Drawing for the job (mm, zero at the part's lowest x, y, z). Give positions to 0.01 mm unless a question says otherwise; leave off trailing zeros. Write each loop counter-clockwise with the first axis right and the second up, starting at its lowest first coordinate (ties: lowest second). Pieces come first, ordered by that corner, then holes.
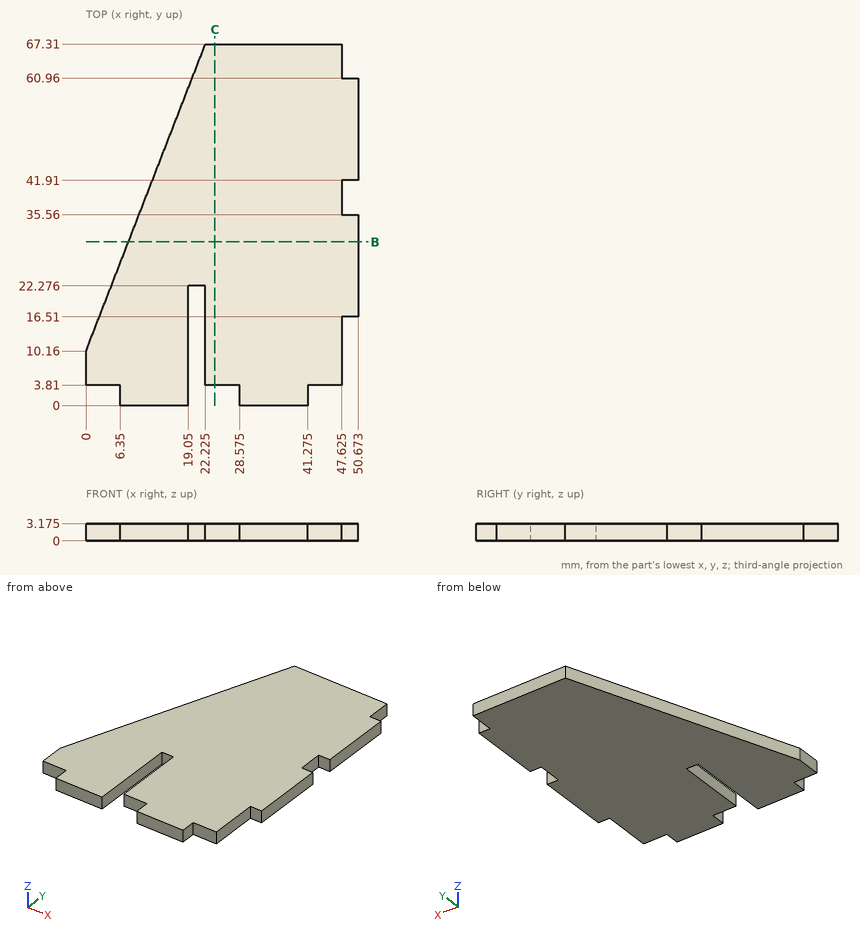
1. Probe probe 1 along Y at (x, z) = (42, 1.9); probe 2 along X at (y, z) = (42, 0.5); probe 3 along X at (y, z) = (41, 2.6) (1 decimal). List the from-to ranges inside material, lowest first.
Calculated:
probe 1: y = 3.81 to 67.31
probe 2: x = 12.38 to 50.67
probe 3: x = 12 to 47.6
2. Slice it at C-C, the plane x = 24. Write the cut outline in (y, z) (3 decimals), and give its area (3 significant figures).
Calculated:
outline: (3.81, 0) - (67.31, 0) - (67.31, 3.175) - (3.81, 3.175) - close
area: 202 mm2
3. Slice it at B-B, the plane y = 30.5. Write the cut outline in (x, z) (3 decimals), and give its area (3 significant figures).
Calculated:
outline: (7.91, 0) - (50.673, 0) - (50.673, 3.175) - (7.91, 3.175) - close
area: 136 mm2
4. Pin check, flat tips, straight feed: P1, Ø1.6, axis at y = 12.5, z = 2, coming from the +X side (3 decimals); P2, Ø1.5, axis at x = 49, z = 2, coming from the +Y side; P3, Ø1.6, axis at x = 21, z = 2, coming from the -Y side. Stop position of each tip, or through.
Calculated:
P1: stops at x = 47.625
P2: stops at y = 60.96
P3: stops at y = 22.28
